Drawing for the job (mm, zero at the part's lowest x, y, z). A direction names the side the tool comes from. Round coordinates to 2 decimals unless told otherwise and drop trailing zeros. Loops run counter-clockwise (first coordinate to the right, second up) from the corner with the lowest first, then second, coordinate; pieces in that order, holes last. Notation, with made-up numbers: M 1,25 L 30,25 A37 cw 30,61 Z; hole C -16,-28.5 d8. An arc over 180 degrees is marked long. Use a Markdown table: item, result. Add a question column.
Q1. Cut at D-D (x = 26). Give the cut face in (y, z).
Q2. Cut at C-C (y = 23). Give the cut face in (x, z) (3 decimals), plus the area to 3 significant figures.
Q3. Tool access for the marked faces 1 and 2: list every direction of +Z, -Z, +X, -X, +Y, -Y with a clear straight run to the whole face (end or side of a thin tool).
Q4. Cut at B-B (x = 50). Give the cut face in (y, z) (3 decimals), plus the area to 3 significant figures.
Q5. Probe line 1 (Y direction, x = 13.5, z = 91); line 2 (Z direction, x = 54, y = 11); line 3 (X direction, y = 35, z = 58). List the from-to ranges inside material, lowest first. Write a range as from..to.
Q6. Cut at A-A (z = 50). Give the cut face in (x, y) (3 decimals).
Q7. Pin check, flat tips, straight feed: pin 1 (2 mm diameter, centred on y = 18, z = 50, fed in from -X) (3 decimals); pin 2 (1 mm diameter, centred on x = 60, y = 33.5, fed in from +Z). Stop position of each tip, or through.
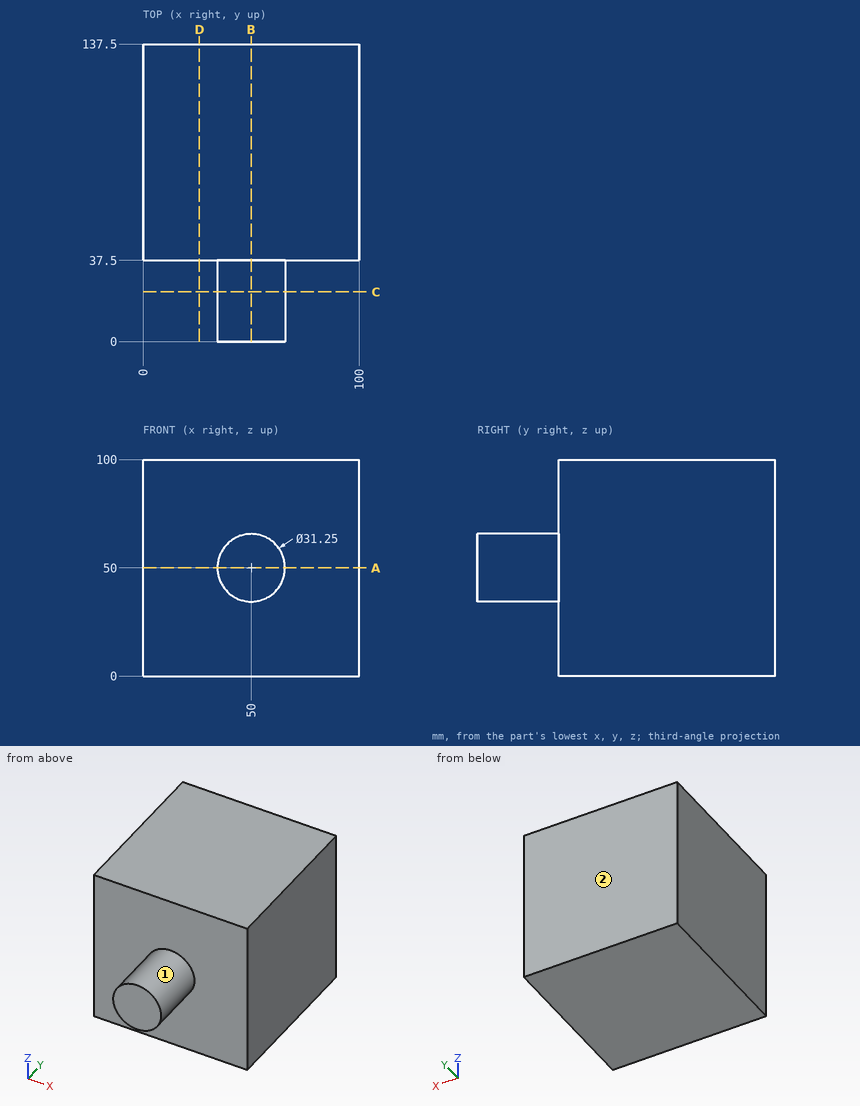
Checked values:
| question | item | result |
|---|---|---|
| 1 | outline | M 37.5,0 L 137.5,0 L 137.5,100 L 37.5,100 Z |
| 2 | outline | C 50,50 d31.25 |
| 2 | area | 767 mm^2 |
| 3 | face 1 | -Y |
| 3 | face 2 | +Z, -Z, +X, -X, +Y |
| 4 | outline | M 0,34.375 L 37.5,34.375 L 37.5,0 L 137.5,0 L 137.5,100 L 37.5,100 L 37.5,65.625 L 0,65.625 Z |
| 4 | area | 11,200 mm^2 |
| 5 | line 1 | y = 37.5..137.5 |
| 5 | line 2 | z = 34.9..65.1 |
| 5 | line 3 | x = 36.58..63.42 |
| 6 | outline | M 0,37.5 L 34.375,37.5 L 34.375,0 L 65.625,0 L 65.625,37.5 L 100,37.5 L 100,137.5 L 0,137.5 Z |
| 7 | pin 1 | stops at x = 34.375 |
| 7 | pin 2 | stops at z = 62.41 |
